from build123d import *

# Parameters (mm, degrees)
SKETCH1_W           = 90
SKETCH1_H           = 90
BOSS_EXTRUDE1_DEPTH = 2.5
SKETCH2_R           = 1.25
BOSS_EXTRUDE2_DEPTH = 1.25


with BuildPart() as part:
    # Sketch1 → Boss-Extrude1 (new body)
    with BuildSketch(Plane.XY):
        Rectangle(SKETCH1_W, SKETCH1_H)
    extrude(amount=BOSS_EXTRUDE1_DEPTH)

    # Sketch2 → Boss-Extrude2 (add)
    with BuildSketch(Plane.XY.offset(2.5)):
        with Locations(Location((-42.5, 42, 0), (0, 0, 180))):
            Circle(SKETCH2_R)
        with Locations(Location((42.5, 42, 0), (0, 0, 180))):
            Circle(SKETCH2_R)
        with Locations(Location((42.5, -42, 0), (0, 0, 180))):
            Circle(SKETCH2_R)
    extrude(amount=BOSS_EXTRUDE2_DEPTH)


solid = part.part
Source: CAD feature listing. Evaluate the final solid. Frame: model axes, mm. A direction names the side the tool comes from. Round coordinates to 2 decimals unless told otherwise and drop trailing zeros. Write each loop counter-clockwise with the first axis right and the second up, starting at its lowest first coordinate (ties: lowest second). Pieces come first, ordered by that corner, then holes. Notation, with made-up numbers: (-8, 48) - (4, 48) arc R12 ccw to (4, 62) - close; hole circle Ø3 at (6.5, 80.25). An arc over 180 degrees is marked (long way). Use CSV: the item, a comma, the result in double quotes. Start each with the question number.
(1) Cut plane B-B, the plane y = 42. Return loops of the section in (x, z), and give its area (3 significant figures).
(2) Cut plane C-C, the plane x = -42.5. Return loops of the section in (y, z), and give its area (3 significant figures).
(3) First-contact query: pin 1 Ø8 at (x, y) = (-34, -8) entering from +Z. Flat tip, straight axial feed; report the tip coordinate or a pass-through.
(4) Cut plane A-A, the plane x = 42.5. Return loops of the section in (y, z).
(5) Cut plane D-D, the plane y = -42. Return loops of the section in (x, z), and give its area (3 significant figures).
(6) Mould query, pull axis Y, two halves, no side actions, for faces 1 (the face through (43.75, 41.95, 3.12)), 2 (the face through (43, -42, 3.75)), 3 (the face through (-1, 45, 1)). Classes: pulls with the +Y half, pulls with the -Y half, needs draft (parallel to the pull), parting line crosses it, or undercut.
(7) Material intervals for probe 1 along Z at (x, y) = (28, 24); probe 2 along X at (y, z) = (41, 3), sorted ascending. Write a range as [from, to].
(8) Set-up query: faces 4 (the face through (-41.25, 41.95, 3.12)), 5 (the face through (-45, -1, 1)). Return all of +Z, -Z, +X, -X, +Y, -Y with unobstructed straight access to the full face (end or side cutting, diameter ignored); none if empty.
Geometry says:
1,outline,"(-45, 0) - (45, 0) - (45, 2.5) - (43.75, 2.5) - (43.75, 3.75) - (41.25, 3.75) - (41.25, 2.5) - (-41.25, 2.5) - (-41.25, 3.75) - (-43.75, 3.75) - (-43.75, 2.5) - (-45, 2.5) - close"
1,area,"231 mm²"
2,outline,"(-45, 0) - (45, 0) - (45, 2.5) - (43.25, 2.5) - (43.25, 3.75) - (40.75, 3.75) - (40.75, 2.5) - (-45, 2.5) - close"
2,area,"228 mm²"
3,pin 1,"z = 2.5"
4,outline,"(-45, 0) - (45, 0) - (45, 2.5) - (43.25, 2.5) - (43.25, 3.75) - (40.75, 3.75) - (40.75, 2.5) - (-40.75, 2.5) - (-40.75, 3.75) - (-43.25, 3.75) - (-43.25, 2.5) - (-45, 2.5) - close"
5,outline,"(-45, 0) - (45, 0) - (45, 2.5) - (43.75, 2.5) - (43.75, 3.75) - (41.25, 3.75) - (41.25, 2.5) - (-45, 2.5) - close"
5,area,"228 mm²"
6,face 1,"undercut"
6,face 2,"needs draft"
6,face 3,"pulls with the +Y half"
7,probe 1,"[0, 2.5]"
7,probe 2,"[-43.25, -41.75], [41.75, 43.25]"
8,face 4,"+Z"
8,face 5,"+Z, -Z, -X, +Y, -Y"
